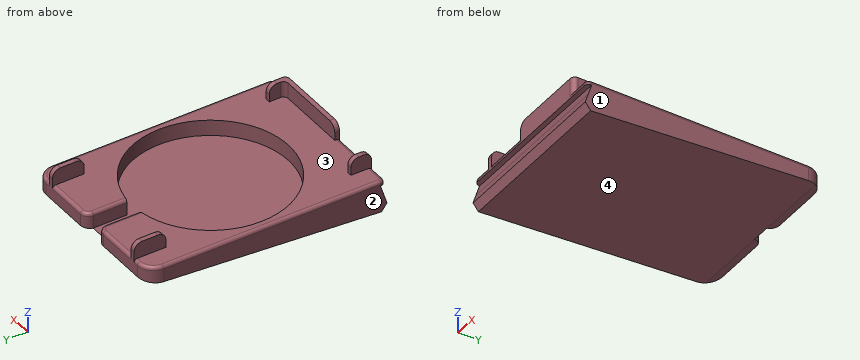
```python
from build123d import *

# Parameters (mm, degrees)
F1_DEPTH      = 10
F3_DEPTH      = 10
F5_DEPTH      = 112.1
F6_DEPTH      = 112.8
F7_DEPTH      = 108
F2_W          = 3
F2_H          = 20
F2_H_2        = 13
F8_DEPTH      = 10
F9_T4_DEPTH   = 34.3846000786
F9_T9_DEPTH   = 34.3846000786
F10_R         = 10
F11_R         = 5
F12_R         = 2
F13_R         = 3
F14_T2_ANGLE  = 90
F14_T4_ANGLE  = 90
F14_T8_DEPTH  = 10.5
F14_T13_DEPTH = 10.5
F15_SIZE      = 5


# Not quite as in the source:
# - a fillet or chamfer that OpenCascade refuses, or shapes differently, is made with other operations: its cross-section is extruded or revolved along the edge and cut away or added
# - a feature names something its author has since deleted; it is built from what else it names


with BuildPart() as f1:
    # F0 (on Top) → F1 (new body)
    with BuildSketch(Plane.XY):
        with BuildLine():
            Line((17.5125259459, 108.1324160099), (-30.4874740541, 108.1324160099))
            Line((-30.4874740541, 108.1324160099), (-30.4874740541, -41.8675839901))
            Line((-30.4874740541, -41.8675839901), (77.5125259459, -41.8675839901))
            Line((77.5125259459, -41.8675839901), (77.5125259459, 108.1324160099))
            Line((77.5125259459, 108.1324160099), (29.5125259459, 108.1324160099))
            Line((29.5125259459, 108.1324160099), (29.5125259459, 82.0155675041))
            ThreePointArc((29.5125259459, 82.0155675041), (23.5125259459, -16.1175839901), (17.5125259459, 82.0155675041))
            Line((17.5125259459, 82.0155675041), (17.5125259459, 108.1324160099))
        make_face()
    extrude(amount=F1_DEPTH)

    # F2 (on face) → F3 (join)
    with BuildSketch(Plane.XY.offset(10)):
        Polygon((13.5125259459, -41.8675839901), (23.5125259459, -41.8675839901), (61.2625259459, -41.8675839901), (61.2625259459, -38.8675839901), (13.5125259459, -38.8675839901), align=None)
    extrude(amount=F3_DEPTH)

    # F4 (on face) → F5 (cut)
    with BuildSketch(Plane.YZ.offset(77.5125259459)):
        Polygon((-38.8675839901, 7), (-41.8675839901, 7), (-41.8675839901, 0), (-41.1420218637, 0), align=None)
    extrude(amount=-F5_DEPTH, mode=Mode.SUBTRACT)

    # F4 (on face) → F6 (cut)
    with BuildSketch(Plane.YZ.offset(77.5125259459)):
        Polygon((108.1324160099, 0), (108.1324160099, 0.6153999214), (103.3824160099, 0), align=None)
    extrude(amount=-F6_DEPTH, mode=Mode.SUBTRACT)

    # F4 (on face) → F7 (join)
    with BuildSketch(Plane.YZ.offset(77.5125259459)):
        Polygon((-38.8675839901, 0), (-41.1420218637, 0), (-44.5225949872, -10.4043342482), (103.3824160099, 0), (-36.5935839901, 0), align=None)
    extrude(amount=-F7_DEPTH)

    # F2 (on face) → F8 (join)
    with BuildSketch(Plane.XY.offset(10)):
        with Locations((-15.7374740541, 98.1324160099)):
            Rectangle(F2_W, F2_H)
        with Locations((62.7625259459, 98.1324160099)):
            Rectangle(F2_W, F2_H)
        with Locations((-15.7374740541, -35.3675839901)):
            Rectangle(F2_W, F2_H_2)
        Polygon((61.2625259459, -38.8675839901), (61.2625259459, -41.8675839901), (64.2625259459, -41.8675839901), (64.2625259459, -28.8675839901), (61.2625259459, -28.8675839901), align=None)
    extrude(amount=F8_DEPTH)

    # F9: fillet of radius 5 on 2 edges, made by hand


with BuildPart() as f9_tool2:
    # F9_s3 → F9_t4 (new body)
    with BuildSketch(Plane.XY.offset(-11.8846000786)):
        with BuildLine():
            ThreePointArc((17.5125259459, 103.1324160099), (16.0480598518, 106.6679499158), (12.5125259459, 108.1324160099))
            Line((12.5125259459, 108.1324160099), (17.5125259459, 108.1324160099))
            Line((17.5125259459, 108.1324160099), (17.5125259459, 103.1324160099))
        make_face()
    extrude(amount=F9_T4_DEPTH)

    split(bisect_by=Plane.XY, keep=Keep.TOP)


with BuildPart() as f1_1:
    add(f1.part)

    # F9_t1: cut F9_tool2
    add(f9_tool2.part, mode=Mode.SUBTRACT)


with BuildPart() as f9_tool7:
    # F9_s8 → F9_t9 (new body)
    with BuildSketch(Plane.XY.offset(-11.8846000786)):
        with BuildLine():
            ThreePointArc((29.5125259459, 103.1324160099), (30.97699204, 106.6679499158), (34.5125259459, 108.1324160099))
            Line((34.5125259459, 108.1324160099), (29.5125259459, 108.1324160099))
            Line((29.5125259459, 108.1324160099), (29.5125259459, 103.1324160099))
        make_face()
    extrude(amount=F9_T9_DEPTH)

    split(bisect_by=Plane.XY, keep=Keep.TOP)


with BuildPart() as f1_2:
    add(f1_1.part)

    # F9_t6: cut F9_tool7
    add(f9_tool7.part, mode=Mode.SUBTRACT)

    # F10
    f10_edges = [f1_2.edges().sort_by_distance(p)[0] for p in [
        (77.512526, 108.132416, 5.3077),
        (-30.487474, 108.132416, 5.3077),
    ]]
    fillet(f10_edges, radius=F10_R)

    # F11
    f11_edges = [f1_2.edges().sort_by_distance(p)[0] for p in [
        (-15.737474, 88.132416, 20),
        (-15.737474, 108.132416, 20),
        (62.762526, 88.132416, 20),
        (62.762526, 108.132416, 20),
        (62.762526, -28.867584, 20),
        (-15.737474, -28.867584, 20),
        (-15.737474, -41.867584, 20),
        (13.512526, -40.367584, 20),
    ]]
    fillet(f11_edges, radius=F11_R)

    # F12
    f12_edges = [f1_2.edges().sort_by_distance(p)[0] for p in [
        (77.512526, 28.132416, 10),
        (-0.362474, -41.867584, 10),
        (70.887526, -41.867584, 10),
        (-23.862474, -41.867584, 10),
        (-30.487474, 28.132416, 10),
        (-27.558542, 105.203484, 10),
        (-18.862474, 108.132416, 10),
        (-0.862474, 108.132416, 10),
        (47.887526, 108.132416, 10),
        (74.583594, 105.203484, 10),
        (65.887526, 108.132416, 10),
        (30.976992, 106.66795, 10),
        (29.512526, 92.573992, 10),
        (17.512526, 92.573992, 10),
        (16.04806, 106.66795, 10),
    ]]
    fillet(f12_edges, radius=F12_R)

    # F13
    f13_edges = [f1_2.edges().sort_by_distance(p)[0] for p in [
        (64.262526, -41.867584, 15),
        (61.262526, -38.867584, 15),
    ]]
    fillet(f13_edges, radius=F13_R)

    # F14: fillet of radius 3 on 2 edges, made by hand

    # F14_s1 → F14_t2 (revolve, cut)
    with BuildSketch(Plane.XZ.offset(38.8675839901)):
        with BuildLine():
            ThreePointArc((-28.4874740541, 10), (-29.9016876165, 9.4142135624), (-30.4874740541, 8))
            Line((-30.4874740541, 8), (-30.4874740541, 10))
            Line((-30.4874740541, 10), (-28.4874740541, 10))
        make_face()
    revolve(axis=Axis((-27.4874740541, -38.8675839901, 10), (0, 0, 1)), revolution_arc=F14_T2_ANGLE, mode=Mode.SUBTRACT)

    # F14_s3 → F14_t4 (revolve, cut)
    with BuildSketch(Plane.YZ.offset(74.5125259459)):
        with BuildLine():
            ThreePointArc((-39.8675839901, 10), (-41.2817975525, 9.4142135624), (-41.8675839901, 8))
            Line((-41.8675839901, 8), (-41.8675839901, 10))
            Line((-41.8675839901, 10), (-39.8675839901, 10))
        make_face()
    revolve(axis=Axis((74.5125259459, -38.8675839901, 10), (0, 0, 1)), revolution_arc=F14_T4_ANGLE, mode=Mode.SUBTRACT)


with BuildPart() as f14_tool6:
    # F14_s7 → F14_t8 (new body)
    with BuildSketch(Plane.XY.offset(-0.5)):
        with BuildLine():
            ThreePointArc((74.5125259459, -41.8675839901), (76.6338462895, -40.9889043337), (77.5125259459, -38.8675839901))
            Line((77.5125259459, -38.8675839901), (77.5125259459, -41.8675839901))
            Line((77.5125259459, -41.8675839901), (74.5125259459, -41.8675839901))
        make_face()
    extrude(amount=F14_T8_DEPTH)

    split(bisect_by=Plane(origin=(0, -37.2133083672, 12.0913368505), x_dir=(1, 0, 0), z_dir=(0, -0.9510565163, 0.3090169944)), keep=Keep.TOP)


with BuildPart() as f1_3:
    add(f1_2.part)

    # F14_t5: cut F14_tool6
    add(f14_tool6.part, mode=Mode.SUBTRACT)


with BuildPart() as f14_tool11:
    # F14_s12 → F14_t13 (new body)
    with BuildSketch(Plane.XY.offset(-0.5)):
        with BuildLine():
            ThreePointArc((-27.4874740541, -41.8675839901), (-29.6087943977, -40.9889043337), (-30.4874740541, -38.8675839901))
            Line((-30.4874740541, -38.8675839901), (-30.4874740541, -41.8675839901))
            Line((-30.4874740541, -41.8675839901), (-27.4874740541, -41.8675839901))
        make_face()
    extrude(amount=F14_T13_DEPTH)

    split(bisect_by=Plane(origin=(0, -37.2133083672, 12.0913368505), x_dir=(1, 0, 0), z_dir=(0, -0.9510565163, 0.3090169944)), keep=Keep.TOP)


with BuildPart() as f1_4:
    add(f1_3.part)

    # F14_t10: cut F14_tool11
    add(f14_tool11.part, mode=Mode.SUBTRACT)

    # F15
    f15_edges = [f1_4.edges().sort_by_distance(p)[0] for p in [
        (23.512526, -44.522595, -10.404334),
    ]]
    chamfer(f15_edges, length=F15_SIZE)


solid = f1_4.part
```
Check sheet for the modelled part. Datum: model origin and axes. Units: mm. Face numbers are marked on the shaded views. Coordinates: 2 decimals unless noted, no trailing zeros. Order: outer loops, then holes, each group sorted by start corner. A loop starts at its lowest first (then second) coordinate and runs counter-clockwise, first axis right, second up. Notation, with made-up numbers: (75.25, 61) -> (114.25, 61) arc R28 cw to (114.25, 81) -> close; hole circle Ø7 at (-39.75, 49.25). An arc over 180 degrees is marked (long way). Write each question's results on one line, items separated by ' | '. Start each with the question number.
1) Section check C-C (z = -4). Enter the section's corners in (x, y).
2) Draft check along X on the marked faces 1, 2, 3 and 4. Enter one of: pulls with the +X half, pulls with the -X half, needs draft (parallel to the pull), parting line crosses it, or undercut.
3) Section check A-A (x = 20.5). Enter the section's corners in (y, z).
4) Material ranges on line 1 along Y through (x, z) = (-15.5, 11.5); line 2 along Y through (x, z) = (32, 18.5); line 3 along Y through (x, z) = (68.5, 8.5), recorded low to high.
5) Depth check by flat-ended pin: pin 1 (3.5 mm diameter, centred on y = -32.5, z = 16, fed in from -X); pin 2 (1 mm diameter, centred on x = 60, z = 16.5, fed in from +Y); pin 3 (10 mm diameter, centred on x = -0.5, y = 23.5, fed in from +Z). Enter the tip coordinate at first touch or a pass-through.
6) Section check B-B (y = 17.5). Enter the section's corners in (x, z), and give its area (3 significant figures).
7) Section check D-D (x = -3). Enter the section's corners in (y, z), and give its area (3 significant figures).
Checked values:
1) outline: (-30.49, -42.44) -> (77.51, -42.44) -> (77.51, 46.52) -> (-30.49, 46.52) -> close
2) face 1: pulls with the +X half | face 2: pulls with the -X half | face 3: undercut | face 4: needs draft
3) outline: (-42.98, -5.65) -> (-39.53, -10.05) -> (103.38, 0) -> (-16.03, 0) -> (-16.03, 10) -> (-38.87, 10) -> (-38.87, 20) -> (-41.87, 20) -> (-41.87, 7) -> (-38.87, 7) -> close
4) line 1: -41.87 to -28.87, 88.13 to 108.13 | line 2: -41.87 to -38.87 | line 3: -41.8 to 13.09, 53.17 to 108.02
5) pin 1: x = -17.24 | pin 2: y = -37.87 | pin 3: z = 0
6) outline: (-30.49, -6.04) -> (77.51, -6.04) -> (77.51, 8) arc R2 ccw to (75.51, 10) -> (70.22, 10) -> (70.22, 0) -> (-23.19, 0) -> (-23.19, 10) -> (-28.49, 10) arc R2 ccw to (-30.49, 8) -> close | area: 797 mm²
7) outline: (-42.98, -5.65) -> (-39.53, -10.05) -> (103.38, 0) -> (108.13, 0.62) -> (108.13, 8) arc R2 ccw to (106.13, 10) -> (74.64, 10) -> (74.64, 0) -> (-8.37, 0) -> (-8.37, 10) -> (-39.87, 10) arc R2 ccw to (-41.87, 8) -> (-41.87, 7) -> (-38.87, 7) -> close | area: 1,390 mm²
